```python
from build123d import *

# Parameters (mm, degrees)
F1_DEPTH = 5.334


with BuildPart() as f1:
    # F0 (on Front) → F1 (new body)
    with BuildSketch(Plane.XZ):
        Polygon((-28.434427, -29.588092), (-28.298704, -24.837712), (-24.091221, -24.837712), (-24.091221, -29.316641), (-19.06939, -29.316641), (-19.06939, -34.745649), (-7.532748, -34.745649), (-7.532748, -24.29481), (1.560839, -24.29481), (1.560839, -34.609925), (12.147406, -34.609925), (12.147406, -29.180918), (17.304963, -29.180918), (17.304963, -24.430534), (21.783892, -24.430534), (21.783892, -29.723817), (26.67, -29.723817), (26.67, -34.609925), (32.234732, -34.609925), (32.234732, 6.107633), (28.027251, 6.107633), (28.027251, 21.580307), (21.919617, 21.580307), (21.919617, 27.009314), (16.626336, 27.009314), (16.626336, 31.216795), (6.989847, 31.216795), (6.989847, 36.510076), (-13.640381, 36.510076), (-13.640381, 31.623971), (-23.819771, 31.623971), (-23.819771, 26.466411), (-28.841604, 26.466411), (-28.841604, 21.580307), (-34.134887, 21.580307), (-34.134887, 6.379084), (-38.749542, 6.379084), (-38.749542, -34.881376), (-33.049084, -34.881376), (-33.049084, -29.588092), align=None)
        Polygon((-18.79794, 21.580307), (-18.119313, 21.580307), (-7.939924, 21.580307), (-7.939924, 16.558474), (-3.596718, 16.558474), (-3.596718, 11.104424), (-3.596718, 1.357252), (-8.211374, 1.357252), (-8.211374, 1.016588), (-8.211374, -3.66458), (-18.526489, -3.66458), (-18.526489, 1.357252), (-23.819771, 1.357252), (-23.819771, 16.151298), (-18.79794, 16.151298), align=None, mode=Mode.SUBTRACT)
        Polygon((6.521792, 1.090871), (6.521792, 15.899813), (6.521792, 16.182272), (11.606061, 16.182272), (11.606061, 21.266542), (21.976355, 21.266542), (21.976355, 16.222624), (26.939571, 16.222624), (26.939571, 11.232948), (26.939571, 0.929466), (22.016706, 0.929466), (22.016706, -4.195155), (11.525358, -4.195155), (11.525358, 1.090871), align=None, mode=Mode.SUBTRACT)
        Polygon((-7.939924, 21.580307), (-18.119313, 21.580307), (-18.79794, 21.580307), (-18.79794, 16.151298), (-23.819771, 16.151298), (-23.819771, 1.357252), (-18.526489, 1.357252), (-18.526489, -3.66458), (-8.211374, -3.66458), (-8.211374, 1.016588), (-13.341749, 1.016588), (-13.341749, 11.104424), (-3.596718, 11.104424), (-3.596718, 16.558474), (-7.939924, 16.558474), align=None)
        Polygon((6.521792, 16.182272), (6.521792, 15.899813), (6.521792, 1.090871), (11.525358, 1.090871), (11.525358, -4.195155), (22.016706, -4.195155), (22.016706, 0.929466), (16.504878, 0.929466), (16.504878, 11.232948), (26.939571, 11.232948), (26.939571, 16.222624), (21.976355, 16.222624), (21.976355, 21.266542), (11.606061, 21.266542), (11.606061, 16.182272), align=None)
    extrude(amount=F1_DEPTH)


solid = f1.part
```
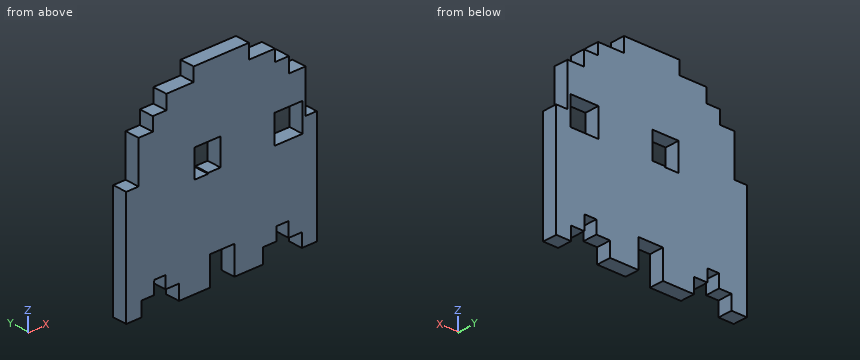
Geometry check sheet. Reference: the model listing, model coordinates, mm. Coordinates: 2 decimals unless noted, no trailing zeros. Order: outer loops, then holes, each group sorted by start corner. A loop starts at its lowest first (then second) coordinate and runs counter-clockwise, first axis right, second up. Notation, with made-up numbers: (-39, -13) - (-33, -13) arc R30 cw to (-33, 22) - close; hole circle Ø1 at (24.5, 76.25). An arc over 180 degrees is marked (long way). Answer in a Markdown table with one row per item. Add a question column.
1. Section check B-B (z = 9). Enter the section's corners in (x, y).
2. Section check D-D (x = -27). Enter the section's corners in (y, z).
3. Material ranges on L1, parallel to X at y = -3.3, z = -25; L2, parallel to X at y = -4.8, z = 4.5; L3, parallel to Z at x = -9, y = -3, recorded low to high. Write a range as [from, to].
4. Gauge pin test, flat ends, axial feed: pin 1 Ø2 at (x, y) = (22.5, -4.5) entering from -Z; pin 2 Ø1.5 at (y, z) = (-1.5, 15.5) entering from +X; pin 3 Ø1.6 at (x, y) = (-1.5, -2.5) entering from -Z. Record the tip position at first contact, or that the pin passes through.
5. Section check C-C (y = -3.95). Give the number of separate pieces and of enclosed holes in the cut face, plus the area to 3 significant figures.
6. Section check A-A (x = 20.5). Enter the section's corners in (y, z).
Data:
| question | item | result |
|---|---|---|
| 1 | outline | (-34.13, -5.33) - (-13.34, -5.33) - (-13.34, 0) - (-34.13, 0) - close; (-3.6, -5.33) - (16.5, -5.33) - (16.5, 0) - (-3.6, 0) - close; (26.94, -5.33) - (28.03, -5.33) - (28.03, 0) - (26.94, 0) - close |
| 2 | outline | (-5.33, -24.84) - (0, -24.84) - (0, 26.47) - (-5.33, 26.47) - close |
| 3 | L1 | x = [-38.75, -28.3], [-24.09, -7.53], [1.56, 17.3], [21.78, 32.23] |
| 3 | L2 | x = [-38.75, -13.34], [-3.6, 16.5], [26.94, 32.23] |
| 3 | L3 | z = [-34.75, 1.02], [11.1, 36.51] |
| 4 | pin 1 | stops at z = -29.72 |
| 4 | pin 2 | stops at x = 28.03 |
| 4 | pin 3 | stops at z = -24.29 |
| 5 | separate pieces | 1 |
| 5 | enclosed holes | 2 |
| 5 | area | 3,930 mm² |
| 6 | outline | (-5.33, -24.43) - (0, -24.43) - (0, 0.93) - (-5.33, 0.93) - close; (-5.33, 11.23) - (0, 11.23) - (0, 27.01) - (-5.33, 27.01) - close |
